from build123d import *

# Parameters (mm, degrees)
SKETCH_1_R                   = 50
EXTRUDE_1_DEPTH              = 5
HOLE_WIZARD_M2_1_D           = 2.4
HOLE_WIZARD_M2_1_CBORE_D     = 4.2
HOLE_WIZARD_M2_1_CBORE_DEPTH = 1.45
HOLE_WIZARD_M3_2_D           = 3.4
HOLE_WIZARD_M3_2_CBORE_D     = 6.05
HOLE_WIZARD_M3_2_CBORE_DEPTH = 2.2
PATTERN_CIRCULAR_1_COUNT     = 8
SKETCH_6_R                   = 8.5
CUT_EXTRUDE_1_DEPTH          = 71.887234394
SKETCH_7_R                   = 5.4875
CUT_EXTRUDE_2_DEPTH          = 71.887234394
FILLET_1_R                   = 1.5
HOLE_WIZARD_M3_3_D           = 3.4
HOLE_WIZARD_M3_3_CBORE_D     = 6.05
HOLE_WIZARD_M3_3_CBORE_DEPTH = 2.2
SKETCH_12_W                  = 5
SKETCH_12_H                  = 2
CUT_EXTRUDE_4_DEPTH          = 71.887234394
SKETCH_14_W                  = 2
SKETCH_14_H                  = 5
EXTRUDE_2_DEPTH              = 3
FILLET_2_R                   = 1
FILLET_2_OF_MIRROR_2_R       = 1


with BuildPart() as part:
    # ｽｹｯﾁ1 → ﾎﾞｽ - 押し出し1 (new body)
    with BuildSketch(Plane.XY):
        Circle(SKETCH_1_R)
    extrude(amount=EXTRUDE_1_DEPTH)

    # M2 丸平ねじ用座ぐり穴1 (through all)
    with Locations(Plane.XY.offset(5)):
        with Locations((-10.5, 0), (-10.5, -21)):
            hole_wizard_m2_1 = CounterBoreHole(HOLE_WIZARD_M2_1_D / 2, HOLE_WIZARD_M2_1_CBORE_D / 2, HOLE_WIZARD_M2_1_CBORE_DEPTH)

    # ﾐﾗｰ1: M2 丸平ねじ用座ぐり穴1 across plane
    add(hole_wizard_m2_1.mirror(Plane(origin=(0, 0, 0), x_dir=(0, 0, 1), z_dir=(1, 0, 0))), mode=Mode.SUBTRACT)

    # M3 丸平ねじ用座ぐり穴2 (through all)
    with Locations(Plane.XY.offset(5)):
        with Locations((46, 0)):
            hole_wizard_m3_2 = CounterBoreHole(HOLE_WIZARD_M3_2_D / 2, HOLE_WIZARD_M3_2_CBORE_D / 2, HOLE_WIZARD_M3_2_CBORE_DEPTH)

    # 円形ﾊﾟﾀｰﾝ1: M3 丸平ねじ用座ぐり穴2 ×8 about axis
    pattern_circular_1_axis = Axis((0, 0, 0), (0, 0, 1))
    for i in range(1, PATTERN_CIRCULAR_1_COUNT):
        add(hole_wizard_m3_2.rotate(pattern_circular_1_axis, i * 360 / PATTERN_CIRCULAR_1_COUNT), mode=Mode.SUBTRACT)

    # ｽｹｯﾁ6 → ｶｯﾄ - 押し出し1 (cut, through all)
    with BuildSketch(Plane.XY.offset(5)):
        Circle(SKETCH_6_R)
    extrude(amount=-CUT_EXTRUDE_1_DEPTH, mode=Mode.SUBTRACT)

    # ｽｹｯﾁ7 → ｶｯﾄ - 押し出し2 (cut, through all)
    with BuildSketch(Plane.XY.offset(5)):
        with Locations((0, -35.4875)):
            Circle(SKETCH_7_R)
    extrude(amount=-CUT_EXTRUDE_2_DEPTH, mode=Mode.SUBTRACT)

    # ﾌｨﾚｯﾄ1
    fillet_1_edges = [part.edges().sort_by_distance(p)[0] for p in [
        (-5.4875, -35.4875, 0),
        (-5.4875, -35.4875, 5),
    ]]
    fillet(fillet_1_edges, radius=FILLET_1_R)

    # M3 丸平ねじ用座ぐり穴3 (through all)
    with Locations(Plane.XY.offset(5)):
        with Locations((22, -2), (22, -12), (-33, -12)):
            CounterBoreHole(HOLE_WIZARD_M3_3_D / 2, HOLE_WIZARD_M3_3_CBORE_D / 2, HOLE_WIZARD_M3_3_CBORE_DEPTH)

    # ｽｹｯﾁ12 → ｶｯﾄ - 押し出し4 (cut, through all)
    with BuildSketch(Plane(origin=(0, 0, 0), x_dir=(-1, 0, 0), z_dir=(0, 0, -1))):
        with Locations((16.5, 35)):
            Rectangle(SKETCH_12_W, SKETCH_12_H)
        with Locations((16.5, 10.5)):
            Rectangle(SKETCH_12_W, SKETCH_12_H)
    cut_extrude_4 = extrude(amount=-CUT_EXTRUDE_4_DEPTH, mode=Mode.SUBTRACT)

    # ｽｹｯﾁ14 → ﾎﾞｽ - 押し出し2 (add)
    with BuildSketch(Plane(origin=(0, 0, 0), x_dir=(-1, 0, 0), z_dir=(0, 0, -1))):
        with Locations((25, 29.5)):
            Rectangle(SKETCH_14_W, SKETCH_14_H)
        with Locations((25, 16)):
            Rectangle(SKETCH_14_W, SKETCH_14_H)
    extrude_2 = extrude(amount=EXTRUDE_2_DEPTH)

    # ﾌｨﾚｯﾄ2
    fillet_2_edges = [part.edges().sort_by_distance(p)[0] for p in [
        (-26, 29.5, 0),
        (-26, 16, 0),
    ]]
    fillet(fillet_2_edges, radius=FILLET_2_R)

    # ﾐﾗｰ2: ｶｯﾄ - 押し出し4, ﾎﾞｽ - 押し出し2 across plane
    add(cut_extrude_4.mirror(Plane(origin=(0, 0, 0), x_dir=(0, 0, 1), z_dir=(1, 0, 0))), mode=Mode.SUBTRACT)
    add(extrude_2.mirror(Plane(origin=(0, 0, 0), x_dir=(0, 0, 1), z_dir=(1, 0, 0))))

    # ﾌｨﾚｯﾄ2 of ﾐﾗｰ2
    fillet_2_of_mirror_2_edges = [part.edges().sort_by_distance(p)[0] for p in [
        (26, 29.5, 0),
        (26, 16, 0),
    ]]
    fillet(fillet_2_of_mirror_2_edges, radius=FILLET_2_OF_MIRROR_2_R)


solid = part.part
Could you check a few things on this model? Use its own coordinates, in mm. A direction names the side the tool comes from. Coordinates: 2 decimals unless noted, no trailing zeros. Write each loop counter-clockwise with the first axis right and the second up, starting at its lowest first coordinate (ties: lowest second). Pieces come first, ordered by that corner, then holes. Notation, with made-up numbers: (-39, 88) - (-22, 88) arc R6 cw to (-22, 95) - close; hole circle Ø5 at (78, 46). An arc over 180 degrees is marked (long way). Put each result on its own line as item: value. Start each with the question number.
Q1. I want a section at A-A on x = 46. Write out the boundary of the cut face in (y, z) (3 decimals).
Q2. Thinking about a two-plate mould opening in Y: for faces 3 (the flat face through (-25, 13.5, -1)), 4 (the flat face through (-10.5, -22.4, 3.55)), which applies, pulls with the +Y half, pulls with the -Y half, needs draft (parallel to the pull), parting line crosses it, or undercut?
Q3. I want a section at B-B on y = -12. Write out the boundary of the cut face in (x, z) (3 decimals).
Q4. Please list where these lines run through material, in increasing order: L1, parallel to Y at x = 24.5, z = -1; L2, parallel to X at y = -4.5, z = 3.25; L3, parallel to Y at x = -30.5, z = 4.5.
Q5. I want a section at D-D on x = -33. Write out the boundary of the cut face in (y, z) (3 decimals).
Q6. Which directions (+Z, -Z, +X, -X, +Y, -Y) give clear straight access to the entire face, cutting with the end or side of a thin tool? Please do faces 1 (the flat face through (9, 0, 3.55)), 2 (the flat face through (16, 11.5, 2)).
Q7. I'm going to push flat-ended pins straight in: P1, Ø3, axis at y = 25.5, z = 1, coming from the -X side; P2, Ø4, axis at y = 15.5, z = 3.5, coming from the +X side; P3, Ø3.5, axis at x = 32.53, y = -32.53, coming from the -Z side; P4, Ø1.9, axis at x = -10.5, y = -21, coming from the +Z side. Where does each tip first touch, or does it pass through?
Checks:
1. outline: (-19.596, 0) - (-1.7, 0) - (-1.7, 2.8) - (-3.025, 2.8) - (-3.025, 5) - (-19.596, 5) - close; (1.7, 0) - (19.596, 0) - (19.596, 5) - (3.025, 5) - (3.025, 2.8) - (1.7, 2.8) - close
2. face 3: pulls with the -Y half
2. face 4: undercut
3. outline: (-48.539, 0) - (-34.7, 0) - (-34.7, 2.8) - (-36.025, 2.8) - (-36.025, 5) - (-48.539, 5) - close; (-31.3, 0) - (20.3, 0) - (20.3, 2.8) - (18.975, 2.8) - (18.975, 5) - (-29.975, 5) - (-29.975, 2.8) - (-31.3, 2.8) - close; (23.7, 0) - (48.539, 0) - (48.539, 5) - (25.025, 5) - (25.025, 2.8) - (23.7, 2.8) - close
4. L1: 13.5 to 18.5, 27 to 32
4. L2: -49.8 to -7.21, 7.21 to 20.3, 23.7 to 49.8
4. L3: -39.62 to -34.77, -30.28 to -13.7, -10.3 to 30.28, 34.77 to 39.62
5. outline: (-37.563, 0) - (-34.16, 0) - (-34.16, 2.8) - (-35.515, 2.8) - (-35.515, 5) - (-37.563, 5) - close; (-30.894, 0) - (-13.7, 0) - (-13.7, 2.8) - (-15.025, 2.8) - (-15.025, 5) - (-29.539, 5) - (-29.539, 2.8) - (-30.894, 2.8) - close; (-10.3, 0) - (30.894, 0) - (30.894, 2.8) - (29.539, 2.8) - (29.539, 5) - (-8.975, 5) - (-8.975, 2.8) - (-10.3, 2.8) - close; (34.16, 0) - (37.563, 0) - (37.563, 5) - (35.515, 5) - (35.515, 2.8) - (34.16, 2.8) - close
6. face 1: +Z
6. face 2: +Z, -Z
7. P1: x = -43.86
7. P2: x = 48.14
7. P3: z = 0
7. P4: through
